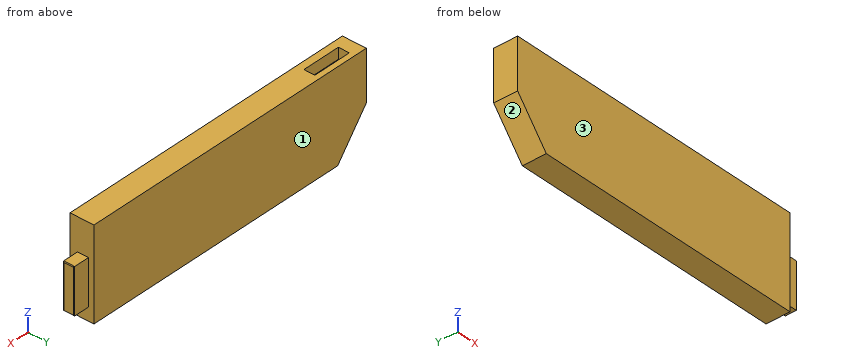
```python
from build123d import *

# Parameters (mm, degrees)
F1_DEPTH      = 5.08
F1_DEPTH_BACK = 4.318
F2_W          = 4.318
F2_H          = 17.78
F3_DEPTH      = 6.35
F4_W          = 15.24
F4_H          = 4.318
F5_DEPTH      = 4.318
F6_SIZE       = 0.254


with BuildPart() as f1:
    # F0 (on Front) → F1 (new body, two sides)
    with BuildSketch(Plane.XZ) as f1_sk:
        Polygon((0, -35.56), (0, 0), (-120.645046, 0), (-120.645046, -19.697705), (-107.945046, -35.56), align=None)
    extrude(amount=F1_DEPTH)
    extrude(f1_sk.sketch, amount=-F1_DEPTH_BACK)

    # F2 (on face) → F3 (join)
    with BuildSketch(Plane.YZ):
        with Locations((0, -21.59)):
            Rectangle(F2_W, F2_H)
    extrude(amount=F3_DEPTH)

    # F4 (on face) → F5 (cut)
    with BuildSketch(Plane.XY):
        with Locations((-107.945046, 0)):
            Rectangle(F4_W, F4_H)
    extrude(amount=-F5_DEPTH, mode=Mode.SUBTRACT)

    # F6
    f6_edges = [f1.edges().sort_by_distance(p)[0] for p in [
        (6.35, 0, -12.7),
        (6.35, -2.159, -21.59),
        (6.35, 0, -30.48),
        (6.35, 2.159, -21.59),
    ]]
    chamfer(f6_edges, length=F6_SIZE)


solid = f1.part
```
The model under review builds one solid part; all positions refer to its coordinate system, in mm. Face numbers are marked on the shaded views. Give positions to 0.01 mm unless a question says otherwise; leave off trailing zeros. Order: outer loops, then holes, each group sorted by start corner. A loop starts at its lowest first (then second) coordinate and runs counter-clockwise, first axis right, second up. Notation, with made-up numbers: (8.25, 66) - (58.25, 66) arc R26 ccw to (58.25, 83) - close; hole circle Ø11 at (-39.5, 39.25). An arc over 180 degrees is marked (long way). Use CSV: the item, a comma, the result in double quotes. Start each with the question number.
Q1. We need section B-B, the plane y = -0.75. Write out the cut boundary in (x, z), and give its area (3 significant figures).
Q2. We need section D-D, the plane z = -22.5. Write out the cut boundary in (x, y) (3 decimals).
Q3. Clearance check with flat-ended pins moving along their axes: pin 1 Ø4.5 at (y, z) = (-2, -10.5) entering from +X; pin 2 Ø3.5 at (x, y) = (4, 0) entering from +Z; pin 3 Ø5 at (y, z) = (2, -5.5) entering from +X. State where each tip first meets the part, or that it passes through.
Q4. We need section A-A, the plane x = -106. Write out the cut boundary in (y, z), and give its area (3 significant figures).
Q5. To check wall thickness, follow line 1 along X through (y, z) = (1.75, -2); line 2 along X through (y, z) = (-3.5, -17); line 3 along X through (y, z) = (-1.5, -28.5). State the ranges of each line that lie inside material, in increasing order. Write a range as [from, to].
Q6. We need section C-C, the plane z = -14.5. Write out the cut boundary in (x, y) (3 decimals), and give its area (3 significant figures).
Q7. The part is to be moulded in two halves that separate along Y. For the marked faces 1, 2 and 3, say which applies: +Y half, -Y half, draft (parallel to the pull), parting line (faces both ways), or undercut.
Outcome:
1,outline,"(-120.65, -19.7) - (-107.95, -35.56) - (0, -35.56) - (0, -30.48) - (6.1, -30.48) - (6.35, -30.23) - (6.35, -12.95) - (6.1, -12.7) - (0, -12.7) - (0, 0) - (-100.33, 0) - (-100.33, -4.32) - (-115.57, -4.32) - (-115.57, 0) - (-120.65, 0) - close"
1,area,"4,240 mm^2"
2,outline,"(-118.401, -5.08) - (0, -5.08) - (0, -2.159) - (6.096, -2.159) - (6.35, -1.905) - (6.35, 1.905) - (6.096, 2.159) - (0, 2.159) - (0, 4.318) - (-118.401, 4.318) - close"
3,pin 1,"stops at x = 6.15"
3,pin 2,"stops at z = -12.7"
3,pin 3,"stops at x = 0"
4,outline,"(-5.08, -35.56) - (4.32, -35.56) - (4.32, 0) - (2.16, 0) - (2.16, -4.32) - (-2.16, -4.32) - (-2.16, 0) - (-5.08, 0) - close"
4,area,"316 mm^2"
5,line 1,"x = [-120.65, -115.57], [-100.33, 0]"
5,line 2,"x = [-120.65, 0]"
5,line 3,"x = [-113.6, 6.35]"
6,outline,"(-120.645, -5.08) - (0, -5.08) - (0, -2.159) - (6.096, -2.159) - (6.35, -1.905) - (6.35, 1.905) - (6.096, 2.159) - (0, 2.159) - (0, 4.318) - (-120.645, 4.318) - close"
6,area,"1,160 mm^2"
7,face 1,"+Y half"
7,face 2,"draft"
7,face 3,"-Y half"
